Model file for the job. Use its own axes, mm. A direction names the side the tool comes from. Give positions to 0.01 mm unless a question says otherwise; leave off trailing zeros. Loops run counter-clockwise (first coordinate to the right, second up) from the corner with the lowest first, then second, coordinate; pieces in that order, holes last. Notation, with made-up numbers: M 47.25,13 L 55.25,13 A21 ccw 55.25,52 Z; hole C 39.5,-16 d6. An arc over 180 degrees is marked long. Use CSV: the item, a comma, the result in double quotes. Start each with the question number.
(1) Tool access for faces 5 (the face through (-14.26, 7.4, 19.38)), 6 (the face through (-2.124, 7.395, -0.035)), 7 (the face through (-5.19, 6.17, -47.54)), 8 (the face through (-7.47, 7.4, 20.42)): list every direction of +Z, -Z, +X, -X, +Y, -Y with a clear straight run to the whole face (end or side of a thin tool).
(2) Two-plate mould, pull along Z, no slides. Class faces 1 (the face through (-11, 7, -47)), 2 (the face through (-6.4, 7.4, -45)), 3 (the face through (-12.866, 7.395, 12.95)), 4 (the face through (-7, 7, 25)): pulls with the +Z half, pulls with the -Z half, needs draft (parallel to the pull), parting line crosses it, or undercut.
(3) Flat gauge pin, fed straight in: P1, Ø2.5, axis at y = 10, z = -48, coming from the -X side. Where does the tip first touch, or does it go through?
(4) Slice it at D-D on z = -41.5. List the corners of the cut face in (x, y), and give its area (3 significant figures).
(5) Slice it at A-A on y = 7.5. List the corners of the cut face in (x, z), and give its area (3 significant figures).
(6) Slice it at B-B on z = 18.5. List the corners of the cut face in (x, y), and give its area (3 significant figures).
(7) Wall check: line 1 along X through (y, z) = (11.5, 16.5); line 2 along Y through (x, z) = (-4.5, -48.9); line 3 along X through (y, z) = (13.25, -11.5). Give the ranges that are in metal, low to high. Write a range as from..to.
(8) Slice it at C-C on y = 3.25. List the corners of the cut face in (x, z), and give its area (3 significant figures).
```python
from build123d import *

# Parameters (mm, degrees)
BOSS_EXTRUDE1_DEPTH = 15
SKETCH3_R           = 1.5
CUT_EXTRUDE2_DEPTH  = 10


with BuildPart() as part:
    # Sketch1 → Boss-Extrude1 (new body)
    with BuildSketch(Plane(origin=(0, 0, 0), x_dir=(1, 0, 0), z_dir=(0, 1, 0))):
        with BuildLine():
            Line((-2, 0.727940469), (-2, 30))
            Line((-2, 30), (-2, 45))
            Line((-2, 45), (-11, 45))
            Line((-11, 45), (-11, 50))
            Line((-11, 50), (2, 50))
            Line((2, 50), (2, 30))
            Line((2, 30), (2, 0.263304995))
            ThreePointArc((2, 0.263304995), (1.982889723, 0.002252611), (1.931851653, -0.254333095))
            Line((1.931851653, -0.254333095), (-4.698729811, -25))
            Line((-4.698729811, -25), (-8.698729811, -25))
            Line((-8.698729811, -25), (-6.211472263, -15.717428462))
            ThreePointArc((-6.211472263, -15.717428462), (-7.219826689, -13.425768705), (-9.675412802, -13.914215152))
            Line((-9.675412802, -13.914215152), (-18.977490779, -25))
            Line((-18.977490779, -25), (-22.977490779, -25))
            Line((-22.977490779, -25), (-2.467911114, -0.557634751))
            ThreePointArc((-2.467911114, -0.557634751), (-2.120614758, 0.043900182), (-2, 0.727940469))
        make_face()
    extrude(amount=BOSS_EXTRUDE1_DEPTH)

    # Sketch3 → Cut-Extrude2 (cut)
    with BuildSketch(Plane(origin=(0, 0, -50), x_dir=(-1, 0, 0), z_dir=(0, 0, -1))):
        with Locations((4.5, 7.5)):
            Circle(SKETCH3_R)
    extrude(amount=-CUT_EXTRUDE2_DEPTH, mode=Mode.SUBTRACT)


solid = part.part
```
Reply:
1,face 5,"+Z, +Y, -Y"
1,face 6,"-X, +Y, -Y"
1,face 7,"-Z"
1,face 8,"+Y, -Y"
2,face 1,"needs draft"
2,face 2,"undercut"
2,face 3,"undercut"
2,face 4,"pulls with the +Z half"
3,P1,"stops at x = -11"
4,outline,"M -2,0 L 2,0 L 2,15 L -2,15 Z"
4,area,"60.0 mm^2"
5,outline,"M -22.98,25 L -2.47,0.56 A2 cw -2,-0.73 L -2,-45 L -3,-45 L -3,-50 L 2,-50 L 2,-0.26 A2 ccw 1.93,0.25 L -4.7,25 L -8.7,25 L -6.21,15.72 A2 cw -9.68,13.91 L -18.98,25 Z; M -11,-50 L -6,-50 L -6,-45 L -11,-45 Z"
5,area,"429 mm^2"
6,outline,"M -17.52,0 L -13.52,0 L -13.52,15 L -17.52,15 Z; M -6.96,0 L -2.96,0 L -2.96,15 L -6.96,15 Z"
6,area,"120 mm^2"
7,line 1,"x = -15.85..-11.85, -6.42..-2.42"
7,line 2,"y = 0..6, 9..15"
7,line 3,"x = -2..2"
8,outline,"M -22.98,25 L -2.47,0.56 A2 cw -2,-0.73 L -2,-45 L -11,-45 L -11,-50 L 2,-50 L 2,-0.26 A2 ccw 1.93,0.25 L -4.7,25 L -8.7,25 L -6.21,15.72 A2 cw -9.68,13.91 L -18.98,25 Z"
8,area,"444 mm^2"
